The model under review builds one solid part; all positions refer to its coordinate system, in mm. A direction names the side the tool comes from. Coordinates: 2 decimals unless noted, no trailing zeros. Order: outer loops, then holes, each group sorted by start corner. A loop starts at its lowest first (then second) coordinate and runs counter-clockwise, first axis right, second up. Notation, with made-up numbers: (-2.75, 68) -> (5.25, 68) arc R38 ccw to (5.25, 107) -> close; hole circle Ø2 at (-30, 11.25). An arc over 180 degrees is marked (long way). Put each result on its own line as item: value.
from build123d import *

# Parameters (mm, degrees)
ESQUISSE1_W        = 25
ESQUISSE1_H        = 252
ESQUISSE1_R        = 5
ESQUISSE1_R_2      = 1.5
BOSS_EXTRU_1_DEPTH = 2
ESQUISSE2_W        = 5.4
ESQUISSE2_H        = 13
ESQUISSE2_H_2      = 10.6
BOSS_EXTRU_2_DEPTH = 16


with BuildPart() as part:
    # Esquisse1 → Boss.-Extru.1 (new body)
    with BuildSketch(Plane(origin=(0, 0, 0), x_dir=(1, 0, 0), z_dir=(0, 1, 0))):
        Rectangle(ESQUISSE1_W, ESQUISSE1_H)
        with Locations((-4.5, 105)):
            Circle(ESQUISSE1_R, mode=Mode.SUBTRACT)
        with Locations((6.5, 105)):
            Circle(ESQUISSE1_R_2, mode=Mode.SUBTRACT)
        with Locations((-4.5, 75)):
            Circle(ESQUISSE1_R, mode=Mode.SUBTRACT)
        with Locations((6.5, 75)):
            Circle(ESQUISSE1_R_2, mode=Mode.SUBTRACT)
        with Locations((-4.5, 45)):
            Circle(ESQUISSE1_R, mode=Mode.SUBTRACT)
        with Locations((6.5, 45)):
            Circle(ESQUISSE1_R_2, mode=Mode.SUBTRACT)
        with Locations((-4.5, 15)):
            Circle(ESQUISSE1_R, mode=Mode.SUBTRACT)
        with Locations((6.5, 15)):
            Circle(ESQUISSE1_R_2, mode=Mode.SUBTRACT)
        with Locations((-4.5, -15)):
            Circle(ESQUISSE1_R, mode=Mode.SUBTRACT)
        with Locations((6.5, -15)):
            Circle(ESQUISSE1_R_2, mode=Mode.SUBTRACT)
        with Locations((-4.5, -45)):
            Circle(ESQUISSE1_R, mode=Mode.SUBTRACT)
        with Locations((6.5, -45)):
            Circle(ESQUISSE1_R_2, mode=Mode.SUBTRACT)
        with Locations((-4.5, -75)):
            Circle(ESQUISSE1_R, mode=Mode.SUBTRACT)
        with Locations((6.5, -75)):
            Circle(ESQUISSE1_R_2, mode=Mode.SUBTRACT)
        with Locations((-4.5, -105)):
            Circle(ESQUISSE1_R, mode=Mode.SUBTRACT)
        with Locations((6.5, -105)):
            Circle(ESQUISSE1_R_2, mode=Mode.SUBTRACT)
        with Locations((-4.5, 120)):
            Circle(ESQUISSE1_R_2, mode=Mode.SUBTRACT)
        with Locations((-4.5, 90)):
            Circle(ESQUISSE1_R_2, mode=Mode.SUBTRACT)
        with Locations((-4.5, 60)):
            Circle(ESQUISSE1_R_2, mode=Mode.SUBTRACT)
        with Locations((-4.5, 30)):
            Circle(ESQUISSE1_R_2, mode=Mode.SUBTRACT)
        with Locations((-4.5, 0)):
            Circle(ESQUISSE1_R_2, mode=Mode.SUBTRACT)
        with Locations((-4.5, -30)):
            Circle(ESQUISSE1_R_2, mode=Mode.SUBTRACT)
        with Locations((-4.5, -60)):
            Circle(ESQUISSE1_R_2, mode=Mode.SUBTRACT)
        with Locations((-4.5, -90)):
            Circle(ESQUISSE1_R_2, mode=Mode.SUBTRACT)
        with Locations((-4.5, -120)):
            Circle(ESQUISSE1_R_2, mode=Mode.SUBTRACT)
    extrude(amount=BOSS_EXTRU_1_DEPTH)

    # Esquisse2 → Boss.-Extru.2 (add)
    with BuildSketch(Plane.XZ):
        with Locations((4.2, -117.1)):
            Rectangle(ESQUISSE2_W, ESQUISSE2_H)
        with Locations((2.6, 118.3)):
            Rectangle(ESQUISSE2_W, ESQUISSE2_H_2)
    extrude(amount=BOSS_EXTRU_2_DEPTH)


solid = part.part
Item 1: For line 1 (X direction, y = 1.2, z = 75); line 2 (X direction, y = 0.9, z = 60); line 3 (Y direction, x = 2.75, z = 0.5), list the stretches that pass through material, from the lowest coordinate up. Write a range as from..to.
Answers below:
line 1: -12.5..-9.5, 0.5..5, 8..12.5
line 2: -12.5..-6, -3..12.5
line 3: 0..2
Item 2: Consider section A-A on y = -7. Write out the cut boundary in (x, z).
Answers below:
outline: (-0.1, 113) -> (5.3, 113) -> (5.3, 123.6) -> (-0.1, 123.6) -> close; (1.5, -123.6) -> (6.9, -123.6) -> (6.9, -110.6) -> (1.5, -110.6) -> close
Item 3: For pin 1 Ø10 at (x, y) = (5.5, -7.5) entering from +Z; pin 2 Ø4 at (x, z) = (-4.5, -120) entering from -Y; pin 3 Ø4 at (x, z) = (-4.5, -90) entering from +Y; pin 4 Ø6 at (x, y) = (5, -10.5) entering from -Z, all flat-tipped, find the tip position at first contact; note any pin that passes through.
Answers below:
pin 1: z = 123.6
pin 2: y = 0
pin 3: y = 2
pin 4: z = -123.6
Item 4: Consider section B-B on z = 64. Write out the cut boundary in (x, y).
Answers below:
outline: (-12.5, 0) -> (12.5, 0) -> (12.5, 2) -> (-12.5, 2) -> close
Item 5: Mouldability with a two-part tool opening along X and no side actions: class faces 1 (the flat face through (1.5, -8, -117)), 2 (the cylindrical face through (-5.58, 0.99, 109.88)), 3 (the flat face through (4, -8, -123.6)) as +X half, -X half, draft (parallel to the pull), parting line (faces both ways), or undercut.
Answers below:
face 1: -X half
face 2: undercut
face 3: draft
Item 6: For faces 4 (the flat face through (6.9, -8, -117)), 5 (the flat face through (3, -8, 123.6)), 6 (the flat face through (4, -8, -110.6)), list the 3-axis set-ups (+Z, -Z, +X, -X, +Y, -Y) from which the entire face can be reached by the end or side of a thin tool; tool diameter is ignored.
Answers below:
face 4: +Z, -Z, +X, -Y
face 5: +Z, +X, -X, -Y
face 6: +X, -X, -Y
